Work out the finished part from the listing and answer in its coordinate system (mm). A direction names the side the tool comes from. Give positions to 0.01 mm unless a question says otherwise; leave off trailing zeros. Write each loop counter-clockwise with the first axis right and the second up, starting at its lowest first coordinate (ties: lowest second). Pieces come first, ordered by that corner, then holes.
1) Find section A-A (x = -1.25). Determine the outline of the cut face in (y, z), plus the area to 3 significant figures.
2) Find section B-B (z = 2.45). Determine the outline of the cut face in (x, y), plus the area to 3 significant figures.
3) Find section C-C (y = -18.5). Determine the outline of the cut face in (x, z).
4) A tool of negligible diameter and unlimited length cuts with its end or side. For faces 1 (the face through (2, -2, 2)), 2 (the face through (-7, -5, 0)), from which of +Z, -Z, +X, -X, +Y, -Y can it reach the whole face along a straight path? Write none if from no direction.
5) Given pin 1 Ø1 at (x, z) = (1.5, 2.5) entering from -Y; pin 2 Ø1.5 at (y, z) = (-9.5, 0.5) entering from +X; pin 3 Ø10 at (x, y) = (3.5, -10.5) entering from +Z (1 decimal), each flat-ended and moving along its own axis, determine where each tip first touches the part or whether it passes through.
6) Straight lines are drawn through the part: probe 1 along Y at (x, z) = (8.5, 2); probe 2 along X at (y, z) = (-8, 2.3); probe 3 along Y at (x, z) = (-4.5, 0.45). For each, find the intervals that lie inside material, in ascending order.
```python
from build123d import *

# Parameters (mm, degrees)
F0_W     = 20
F0_H     = 4
F1_DEPTH = 4
F2_W     = 4
F2_H     = 4
F3_DEPTH = 20
F4_R     = 1
F5_R     = 1
F6_R     = 1


with BuildPart() as f1:
    # F0 (on Top) → F1 (new body)
    with BuildSketch(Plane.XY):
        Rectangle(F0_W, F0_H)
    extrude(amount=F1_DEPTH)

    # F2 (on face) → F3 (join)
    with BuildSketch(Plane.XZ.offset(2)):
        with Locations((-8, 2)):
            Rectangle(F2_W, F2_H)
    extrude(amount=F3_DEPTH)

    # F4
    f4_edges = [f1.edges().sort_by_distance(p)[0] for p in [
        (-10, -10, 4),
    ]]
    fillet(f4_edges, radius=F4_R)

    # F5
    f5_edges = [f1.edges().sort_by_distance(p)[0] for p in [
        (-10, -10, 0),
    ]]
    fillet(f5_edges, radius=F5_R)

    # F6
    f6_edges = [f1.edges().sort_by_distance(p)[0] for p in [
        (0.5, 2, 4),
        (0.5, 2, 0),
    ]]
    fillet(f6_edges, radius=F6_R)


solid = f1.part
```
Results:
1. outline: (-2, 0) - (1, 0) arc R1 ccw to (2, 1) - (2, 3) arc R1 ccw to (1, 4) - (-2, 4) - close
1. area: 15.6 mm2
2. outline: (-10, -22) - (-6, -22) - (-6, -2) - (10, -2) - (10, 2) - (-9, 2) arc R1 ccw to (-10, 1) - close
2. area: 160 mm2
3. outline: (-10, 1) arc R1 ccw to (-9, 0) - (-6, 0) - (-6, 4) - (-9, 4) arc R1 ccw to (-10, 3) - close
4. face 1: +Z, -Z, +X, -Y
4. face 2: -Z, +X, -X, +Y, -Y
5. pin 1: stops at y = -2
5. pin 2: stops at x = -6
5. pin 3: passes through
6. probe 1: y = -2 to 2
6. probe 2: x = -10 to -6
6. probe 3: y = -2 to 1.84
